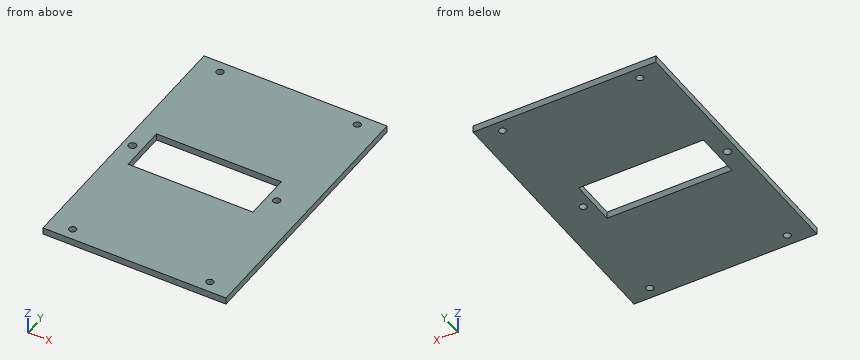
from build123d import *

# Parameters (mm, degrees)
SKETCH_1_W          = 80
SKETCH_1_H          = 117.5
SKETCH_1_W_2        = 35
SKETCH_1_H_2        = 15
EXTRUDE_1_DEPTH     = 3
CUT_EXTRUDE_2_REACH = 144.18
SKETCH_3_R          = 1.55
CUT_EXTRUDE_3_REACH = 144.18
SKETCH_4_R          = 1.55
SKETCH_5_R          = 1.67340685
CUT_EXTRUDE_4_DEPTH = 10
SKETCH_6_W          = 45.612722832
SKETCH_6_H          = 20.743194246
CUT_EXTRUDE_5_DEPTH = 10
SKETCH_7_W          = 3
SKETCH_7_H          = 20.743194246
CUT_EXTRUDE_6_DEPTH = 9


with BuildPart() as part:
    # 草图1 → 凸台-拉伸1 (new body)
    with BuildSketch(Plane.XY):
        with Locations((40, 58.75)):
            Rectangle(SKETCH_1_W, SKETCH_1_H)
        with Locations((40, 58.75)):
            Rectangle(SKETCH_1_W_2, SKETCH_1_H_2, mode=Mode.SUBTRACT)
    extrude(amount=EXTRUDE_1_DEPTH)

    # 草图3 → 切除-拉伸2 (cut, up to next)
    with BuildSketch(Plane.XY.offset(3), mode=Mode.PRIVATE) as cut_extrude_2_sk1:
        with Locations((10, 112.5)):
            Circle(SKETCH_3_R)
    cut_extrude_2_tool1 = extrude(cut_extrude_2_sk1.sketch, amount=-CUT_EXTRUDE_2_REACH, mode=Mode.PRIVATE) & part.part
    # 草图3 → 切除-拉伸2 (cut, up to next)
    with BuildSketch(Plane.XY.offset(3), mode=Mode.PRIVATE) as cut_extrude_2_sk2:
        with Locations((70, 112.5)):
            Circle(SKETCH_3_R)
    cut_extrude_2_tool2 = extrude(cut_extrude_2_sk2.sketch, amount=-CUT_EXTRUDE_2_REACH, mode=Mode.PRIVATE) & part.part
    # 草图3 → 切除-拉伸2 (cut, up to next)
    with BuildSketch(Plane.XY.offset(3), mode=Mode.PRIVATE) as cut_extrude_2_sk3:
        with Locations((70, 5)):
            Circle(SKETCH_3_R)
    cut_extrude_2_tool3 = extrude(cut_extrude_2_sk3.sketch, amount=-CUT_EXTRUDE_2_REACH, mode=Mode.PRIVATE) & part.part
    # 草图3 → 切除-拉伸2 (cut, up to next)
    with BuildSketch(Plane.XY.offset(3), mode=Mode.PRIVATE) as cut_extrude_2_sk4:
        with Locations((10, 5)):
            Circle(SKETCH_3_R)
    cut_extrude_2_tool4 = extrude(cut_extrude_2_sk4.sketch, amount=-CUT_EXTRUDE_2_REACH, mode=Mode.PRIVATE) & part.part
    add(cut_extrude_2_tool1.solids().sort_by_distance((10, 112.5, 3))[0], mode=Mode.SUBTRACT)
    add(cut_extrude_2_tool2.solids().sort_by_distance((70, 112.5, 3))[0], mode=Mode.SUBTRACT)
    add(cut_extrude_2_tool3.solids().sort_by_distance((70, 5, 3))[0], mode=Mode.SUBTRACT)
    add(cut_extrude_2_tool4.solids().sort_by_distance((10, 5, 3))[0], mode=Mode.SUBTRACT)

    # 草图4 → 切除-拉伸3 (cut, up to next)
    with BuildSketch(Plane(origin=(0, 0, 0), x_dir=(-1, 0, 0), z_dir=(0, 0, -1)), mode=Mode.PRIVATE) as cut_extrude_3_sk1:
        with Locations((-67, 58.75)):
            Circle(SKETCH_4_R)
    cut_extrude_3_tool1 = extrude(cut_extrude_3_sk1.sketch, amount=-CUT_EXTRUDE_3_REACH, mode=Mode.PRIVATE) & part.part
    # 草图4 → 切除-拉伸3 (cut, up to next)
    with BuildSketch(Plane(origin=(0, 0, 0), x_dir=(-1, 0, 0), z_dir=(0, 0, -1)), mode=Mode.PRIVATE) as cut_extrude_3_sk2:
        with Locations((-13, 58.75)):
            Circle(SKETCH_4_R)
    cut_extrude_3_tool2 = extrude(cut_extrude_3_sk2.sketch, amount=-CUT_EXTRUDE_3_REACH, mode=Mode.PRIVATE) & part.part
    add(cut_extrude_3_tool1.solids().sort_by_distance((67, 58.75, 0))[0], mode=Mode.SUBTRACT)
    add(cut_extrude_3_tool2.solids().sort_by_distance((13, 58.75, 0))[0], mode=Mode.SUBTRACT)

    # 草图5 → 切除-拉伸4 (cut)
    with BuildSketch(Plane(origin=(0, 0, 0), x_dir=(-1, 0, 0), z_dir=(0, 0, -1))):
        with Locations((-4, 58.576267849)):
            Circle(SKETCH_5_R)
    extrude(amount=-CUT_EXTRUDE_4_DEPTH, mode=Mode.SUBTRACT)

    # 草图6 → 切除-拉伸5 (cut)
    with BuildSketch(Plane.XY.offset(3)):
        with Locations((40, 58.75)):
            Rectangle(SKETCH_6_W, SKETCH_6_H)
    extrude(amount=-CUT_EXTRUDE_5_DEPTH, mode=Mode.SUBTRACT)

    # 草图7 → 切除-拉伸6 (cut)
    with BuildSketch(Plane(origin=(17.193638584, 0, 0), x_dir=(0, 0, -1), z_dir=(1, 0, 0))):
        with Locations((-1.5, 58.75)):
            Rectangle(SKETCH_7_W, SKETCH_7_H)
    extrude(amount=-CUT_EXTRUDE_6_DEPTH, mode=Mode.SUBTRACT)


solid = part.part
Check sheet for the modelled part. Datum: model origin and axes. Units: mm. Round coordinates to 2 decimals unless told otherwise and drop trailing zeros. Loops run counter-clockwise (first coordinate to the right, second up) from the corner with the lowest first, then second, coordinate; pieces in that order, holes last. Notation, with made-up numbers: M 18.5,0 L 30.5,0 A21 ccw 30.5,6 Z; hole C 16.25,2.25 d1. An arc over 180 degrees is marked long. One line per question, with ' | ' between items. Start each with the question number.
Item 1: Scan lines: probe 1 along Y at (x, z) = (10, 1.15); probe 2 along X at (y, z) = (62, 1.2); probe 3 along Y at (x, z) = (61, 2.85). Record each from-to range of solid material in increasing order.
Item 2: Section check D-D (y = 112.5). Record the boundary of the cut face in (x, z), and give its area (3 significant figures).
Item 3: Section check C-C (x = 70). Record the boundary of the cut face in (y, z).
Item 4: Gauge pin test, flat end, axial feed: pin 1 Ø3.5 at (x, y) = (10, 5) entering from +Z. Record the tip position at first contact, or that the pin passes through.
Item 5: Section check A-A (y = 54). Record the boundary of the cut face in (x, z).
Item 6: Section check B-B (x = 60). Record the boundary of the cut face in (y, z), and give its area (3 significant figures).
Worked out:
1) probe 1: 0 to 3.45, 6.55 to 48.38, 69.12 to 110.95, 114.05 to 117.5 | probe 2: 0 to 8.19, 62.81 to 80 | probe 3: 0 to 48.38, 69.12 to 117.5
2) outline: M 0,0 L 8.45,0 L 8.45,3 L 0,3 Z; M 11.55,0 L 68.45,0 L 68.45,3 L 11.55,3 Z; M 71.55,0 L 80,0 L 80,3 L 71.55,3 Z | area: 221 mm^2
3) outline: M 0,0 L 3.45,0 L 3.45,3 L 0,3 Z; M 6.55,0 L 110.95,0 L 110.95,3 L 6.55,3 Z; M 114.05,0 L 117.5,0 L 117.5,3 L 114.05,3 Z
4) pin 1: z = 3
5) outline: M 0,0 L 8.19,0 L 8.19,3 L 0,3 Z; M 62.81,0 L 80,0 L 80,3 L 62.81,3 Z
6) outline: M 0,0 L 48.38,0 L 48.38,3 L 0,3 Z; M 69.12,0 L 117.5,0 L 117.5,3 L 69.12,3 Z | area: 290 mm^2
